```python
from build123d import *

# Parameters (mm, degrees)
BOSS_EXTRUDE1_DEPTH                          = 3
FILLET1_R                                    = 1
CSK_FOR_M4_COUNTERSUNK_FLAT_HEAD_SCR_2_COUNT = 2
CSK_FOR_M4_COUNTERSUNK_FLAT_HEAD_SCR_2_PITCH = 22.627416998
SKETCH4_R                                    = 5
BOSS_EXTRUDE2_DEPTH                          = 5
SKETCH5_R                                    = 1.45
CUT_EXTRUDE1_DEPTH                           = 9


with BuildPart() as part:
    # Sketch1 → Boss-Extrude1 (new body)
    with BuildSketch(Plane(origin=(0, 0, 0), x_dir=(1, 0, 0), z_dir=(0, 1, 0))):
        with BuildLine():
            Line((-16.535533906, -9.464466094), (-8.485281374, -1.414213562))
            Line((-8.485281374, -1.414213562), (-12.949747468, 3.050252532))
            ThreePointArc((-12.949747468, 3.050252532), (-12.949747468, 12.949747468), (-3.050252532, 12.949747468))
            Line((-3.050252532, 12.949747468), (1.414213562, 8.485281374))
            Line((1.414213562, 8.485281374), (9.464466094, 16.535533906))
            ThreePointArc((9.464466094, 16.535533906), (16.535533906, 16.535533906), (16.535533906, 9.464466094))
            Line((16.535533906, 9.464466094), (8.485281374, 1.414213562))
            Line((8.485281374, 1.414213562), (12.949747468, -3.050252532))
            ThreePointArc((12.949747468, -3.050252532), (12.949747468, -12.949747468), (3.050252532, -12.949747468))
            Line((3.050252532, -12.949747468), (-1.414213562, -8.485281374))
            Line((-1.414213562, -8.485281374), (-9.464466094, -16.535533906))
            ThreePointArc((-9.464466094, -16.535533906), (-16.535533906, -16.535533906), (-16.535533906, -9.464466094))
        make_face()
    extrude(amount=BOSS_EXTRUDE1_DEPTH)

    # Fillet1
    fillet1_edges = [part.edges().sort_by_distance(p)[0] for p in [
        (8.485281374, 1.5, -1.414213562),
        (-1.414213562, 1.5, 8.485281374),
        (-8.485281374, 1.5, 1.414213562),
        (1.414213562, 1.5, -8.485281374),
    ]]
    fillet(fillet1_edges, radius=FILLET1_R)

    # Sketch2 → CSK for M4 Countersunk Flat Head Screw1 (revolve, cut)
    with BuildSketch(Plane(origin=(-8, 3, -8), x_dir=(0, 0, 1), z_dir=(1, 0, 0))):
        Polygon((0, 0), (0, 3), (2.25, 3), (2.25, 2.45), (4.7, 0), align=None)
    csk_for_m4_countersunk_flat_head_screw1 = revolve(axis=Axis((-8, 9.35, -8), (0, -1, 0)), mode=Mode.SUBTRACT)

    # CSK for M4 Countersunk Flat Head Scr 2: CSK for M4 Countersunk Flat Head Screw1 ×2
    with Locations(*[Vector(0.707106781, 0, 0.707106781) * (i * CSK_FOR_M4_COUNTERSUNK_FLAT_HEAD_SCR_2_PITCH) for i in range(1, CSK_FOR_M4_COUNTERSUNK_FLAT_HEAD_SCR_2_COUNT)]):
        add(csk_for_m4_countersunk_flat_head_screw1, mode=Mode.SUBTRACT)

    # Sketch4 → Boss-Extrude2 (add)
    with BuildSketch(Plane(origin=(0, 3, 0), x_dir=(1, 0, 0), z_dir=(0, 1, 0))):
        with Locations((-13, -13)):
            Circle(SKETCH4_R)
        with Locations((13, 13)):
            Circle(SKETCH4_R)
    extrude(amount=BOSS_EXTRUDE2_DEPTH)

    # Sketch5 → Cut-Extrude1 (cut, through all)
    with BuildSketch(Plane(origin=(0, 8, 0), x_dir=(1, 0, 0), z_dir=(0, 1, 0))):
        with Locations((-13, -13)):
            Circle(SKETCH5_R)
        with Locations((13, 13)):
            Circle(SKETCH5_R)
    extrude(amount=-CUT_EXTRUDE1_DEPTH, mode=Mode.SUBTRACT)


solid = part.part
```
The model under review builds one solid part; all positions refer to its coordinate system, in mm. A direction names the side the tool comes from. Round coordinates to 2 decimals unless told otherwise and drop trailing zeros. Loops run counter-clockwise (first coordinate to the right, second up) from the corner with the lowest first, then second, coordinate; pieces in that order, holes last. Notation, with made-up numbers: (-11, -33) -> (27, -33) arc R21 ccw to (27, -21) -> close; hole circle Ø1 at (62.25, -28). An arc over 180 degrees is marked (long way). Answer as a JSON object with one key per item and string values. Group by question number.
1) Mouldability with a two-part tool opening along Z and no side actions: class faces 6 (the face through (-12.915, 1.479, 5.844)), 7 (the face through (-1.4, 1.5, 8.9)), 8 (the face through (-14.2, 8, 11.8)) as released by +Z, released by -Z, zero draft, split by the parting line, or undercut.
2) For pin 1 Ø4 at (x, y) = (-7.5, 2.5) entering from +Z; pin 2 Ø10 at (x, z) = (7, 5) entering from +Y; pin 3 Ø5 at (x, z) = (8, 8) entering from +Y, all flat-tipped, find the tip position at first contact; note any pin that passes through.
3) For line 1 (X direction, y = 5, z = -13); line 2 (Z direction, x = -12, y = 2); line 3 (Z direction, x = 10.5, y = 1.75), list the stretches that pass through material, from the lowest coordinate up. Write a range as [from, to].
4) We need section C-C on x = -16. Write out the cut boundary in (y, z), then the cut area to 3 significant figures.
5) We need section B-B on y = 6.5. Write out the cut boundary in (x, z), then the cut area to 3 significant figures.
6) We need section D-D on z = 0. Write out the cut boundary in (x, y), then the cut area to 3 significant figures.
7) For faces 1 (the face through (5.74, 1.48, -12.81)), 2 (the face through (8.86, 0.28, 10.08)), 3 (the face through (12.915, 1.479, -5.844)), 4 (the face through (-11, 1.5, -1.1)), 5 (the face through (-5.74, 1.48, 12.81)), list the 3-axis set-ups (+Z, -Z, +X, -X, +Y, -Y) from which the entire face can be reached by the end or side of a thin tool; tool diameter is ignored.
8) We need section A-A on y = 1. Write out the cut boundary in (x, z).
Result set:
{
 "1": {"face 6": "undercut", "face 7": "released by +Z", "face 8": "zero draft"},
 "2": {"pin 1": "z = 16.57", "pin 2": "y = 3", "pin 3": "y = 0.8"},
 "3": {"line 1": "[8, 11.55], [14.45, 18]", "line 2": "[-13.74, -2.1], [4.93, 11.95], [14.05, 17.9]", "line 3": "[-17.33, -3.43], [0.6, 5.62], [10.38, 14.54]"},
 "4": {"outline": "(0, 8.93) -> (3, 8.93) -> (3, 9) -> (8, 9) -> (8, 17) -> (0, 17) -> close", "area": "64.2 mm²"},
 "5": {"outline": "circle Ø10 at (-13, 13); circle Ø10 at (13, -13); hole circle Ø2.9 at (-13, 13); hole circle Ø2.9 at (13, -13)", "area": "144 mm²"},
 "6": {"outline": "(-9.9, 0) -> (9.9, 0) -> (9.9, 3) -> (-9.9, 3) -> close", "area": "59.4 mm²"},
 "7": {"face 1": "-Z, +Y, -Y", "face 2": "+Y, -Y", "face 3": "+X, +Y, -Y", "face 4": "-X, +Y, -Y", "face 5": "+Z, +Y, -Y"},
 "8": {"outline": "(-16.54, 9.46) -> (-9.19, 2.12) arc R1 cw to (-9.19, 0.71) -> (-12.95, -3.05) arc R7 ccw to (-3.05, -12.95) -> (0.71, -9.19) arc R1 cw to (2.12, -9.19) -> (9.46, -16.54) arc R5 ccw to (16.54, -9.46) -> (9.19, -2.12) arc R1 cw to (9.19, -0.71) -> (12.95, 3.05) arc R7 ccw to (3.05, 12.95) -> (-0.71, 9.19) arc R1 cw to (-2.12, 9.19) -> (-9.46, 16.54) arc R5 ccw to start; hole circle Ø2.9 at (-13, 13); hole circle Ø5.4 at (-8, -8); hole circle Ø5.4 at (8, 8); hole circle Ø2.9 at (13, -13)"}
}
